Drawing for the job (mm, zero at the part's lowest x, y, z). A direction names the side the tool comes from. Coordinates: 2 decimals unless noted, no trailing zeros. Write each loop counter-clockwise with the first axis right and the second up, starting at its lowest first coordinate (ties: lowest second). Pieces come first, ordered by that corner, then holes. Notation, with made-up numbers: (-20, -23) -> (9, -23) arc R16 ccw to (9, -6) -> close; hole circle Ø8 at (-32.75, 0.5). An arc over 180 degrees is marked (long way). Write item = value, one per line. Start each with the question number.
Q1. Tool access for the marked faces 1 and 2: list every direction of +Z, -Z, +X, -X, +Y, -Y with a clear straight run to the whole face (end or side of a thin tool).
Q2. Pull direction Y, two halves, no side cores. Call the marked faces 3, 4 and 5: released by +Y, released by -Y, zero draft, split by the parting line, or undercut.
Q3. Pin check, flat tips, straight feed: P1, Ø1.6, axis at x = 1.5, y = 4, coming from the +Z side; P2, Ø2, axis at y = 4, z = 3, coming from the -X side; P3, Ø1.5, axis at y = 3, z = 1.5, coming from the +X side; P4, Ø0.7, axis at x = 1, y = 4, coming from the -Z side. Stop position of each tip, or through.
Q4. Probe line 1 (X direction, y = 4.75, z = 4); line 2 (Y direction, x = 4.5, z = 4). List the from-to ranges inside material, lowest first.
Q5. Band-saw the part on A-A, the plane y = 4. List the corners of the cut face in (x, z).
Q6. Band-saw the part on B-B, the plane x = 5.15. List the corners of the cut face in (y, z).
Q7. Band-saw the part on C-C, the plane x = 2.1. List the corners of the cut face in (y, z), plus the area to 3 significant figures.
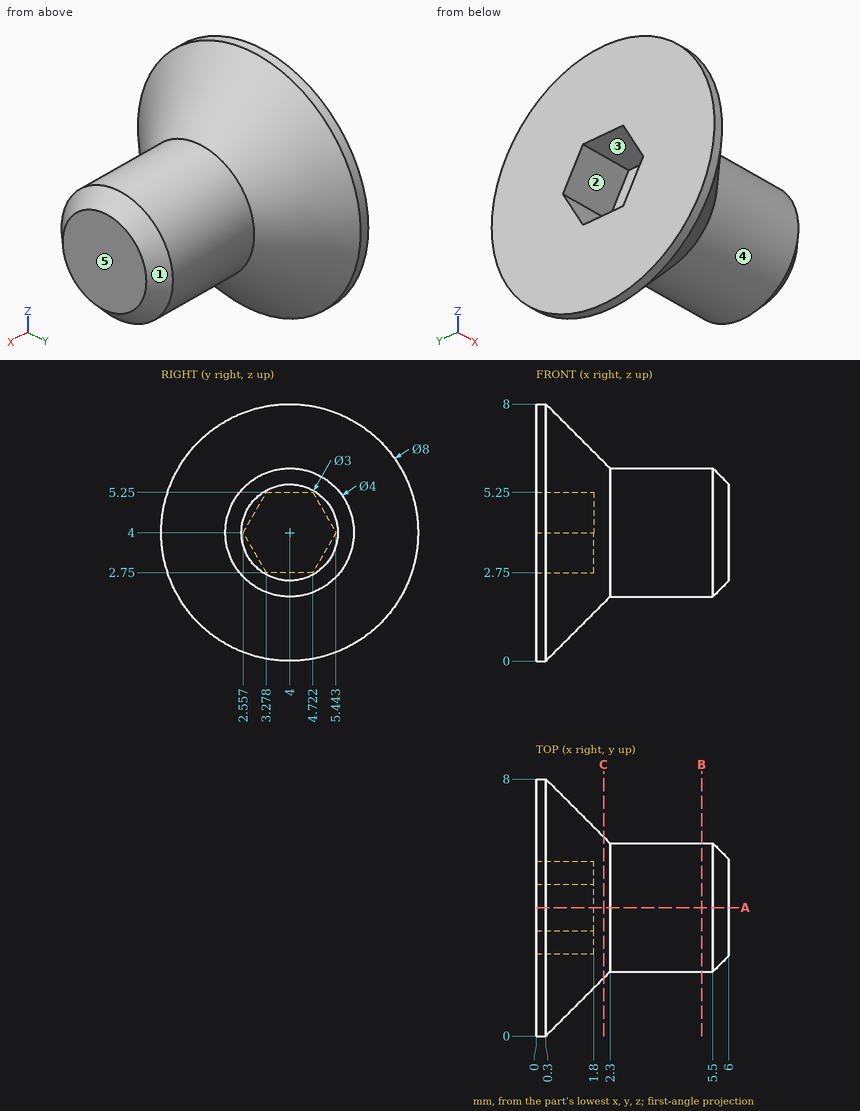
Ans:
q1.face_1 = +X
q1.face_2 = -X
q2.face_3 = undercut
q2.face_4 = split by the parting line
q2.face_5 = zero draft
q3.P1 = 7.6
q3.P2 = 0
q3.P3 = 5.56
q3.P4 = 0.35
q4.line_1 = 1.8 to 6
q4.line_2 = 2 to 6
q5.outline = (0, 0) -> (0.3, 0) -> (2.3, 2) -> (5.5, 2) -> (6, 2.5) -> (6, 5.5) -> (5.5, 6) -> (2.3, 6) -> (0.3, 8) -> (0, 8) -> (0, 5.25) -> (1.8, 5.25) -> (1.8, 2.75) -> (0, 2.75) -> close
q6.outline = circle Ø4 at (4, 4)
q7.outline = circle Ø4.4 at (4, 4)
q7.area = 15.2 mm2
